Can you work these out from the model? Positions are in its coordinate system, mm. A direction names the side the tool comes from. Coordinates: 2 decimals unless noted, no trailing zeros. Order: outer loops, then holes, each group sorted by start corner. A loop starts at its lowest first (then second) coordinate and runs counter-clockwise, first axis right, second up. Notation, with made-up numbers: (26.25, -22) - (55.25, -22) arc R34 ccw to (55.25, 8) - close; hole circle Ø4 at (82.25, -21.5). An arc over 180 degrees is marked (long way). Return JSON: item names as keys, results as strings. Group by question number.
1) Imagine slicing it at C-C (y = -4.75). Write out the boundary of the cut face in (x, z), and give its area (3 significant figures).
2) If I drill on line 1 along Y through (x, z) = (-5.25, -5.5); line 2 along Z through (x, y) = (0, -2.75); line 3 along X through (y, z) = (-4.75, -1.75), over which ranges is the centre line in solid material (lowest first)?
3) If we mould it in two halves opening along X, with no side actions, what happens to faces 4 (the face through (9.4, 1.93, -0.11)), 5 (the face through (-9.43, 1.9, -0.11)), 6 (the face through (-7.5, -1, 0))? For each: pulls with the +X half, pulls with the -X half, needs draft (parallel to the pull), parting line crosses it, or undercut.
4) Imagine slicing it at B-B (x = 1.25). Write out the boundary of the cut face in (y, z).
5) Imagine slicing it at D-D (z = 1.75). Write out the boundary of the cut face in (x, y), and give its area (3 significant figures).
6) Which directions (+Z, -Z, +X, -X, +Y, -Y) give clear straight access to the entire face, cutting with the end or side of a thin tool? Please do faces 1 (the face through (-1, -3, -1.5)), 2 (the face through (1.5, -3, 1)), 3 (the face through (1, -3, -1.5)).
7) For pin 1 Ø2.5 at (y, z) = (-1.5, 0.5) entering from +X; pin 2 Ø0.5 at (x, y) = (1.5, -4.5) entering from +Z; pin 3 Ø0.5 at (y, z) = (-4, 1.5) entering from -X, each with a flat end and sliding along its axis, tell me the tip position at first contact or that it passes through.
8) Imagine slicing it at A-A (y = -1.5). Write out the boundary of the cut face in (x, z), and give its area (3 significant figures).
```python
from build123d import *

# Parameters (mm, degrees)
SKETCH1_W           = 20
SKETCH1_H           = 20
BOSS_EXTRUDE1_DEPTH = 2.5
BOSS_EXTRUDE2_DEPTH = 6
SKETCH3_W           = 2
SKETCH3_H           = 5
BOSS_EXTRUDE3_DEPTH = 3
FILLET1_R           = 2


with BuildPart() as part:
    # Sketch1 → Boss-Extrude1 (new body)
    with BuildSketch(Plane(origin=(0, 2.5, 0), x_dir=(1, 0, 0), z_dir=(0, 1, 0))):
        Rectangle(SKETCH1_W, SKETCH1_H)
    extrude(amount=-BOSS_EXTRUDE1_DEPTH)

    # Sketch2 → Boss-Extrude2 (add)
    with BuildSketch(Plane.XZ):
        with BuildLine():
            Line((-2.015564435, 1.000000009), (-1.000000005, 1.000000009))
            Line((-1.000000005, 1.000000009), (-1.000000005, 2.015564439))
            ThreePointArc((-1.000000005, 2.015564439), (0, 2.250000005), (1.000000005, 2.015564439))
            Line((1.000000005, 2.015564439), (1.000000005, 1.000000009))
            Line((1.000000005, 1.000000009), (2.015564435, 1.000000009))
            ThreePointArc((2.015564435, 1.000000009), (2.25, 5e-09), (2.015564435, -1))
            Line((2.015564435, -1), (1.000000005, -1))
            Line((1.000000005, -1), (1.000000005, -2.01556443))
            ThreePointArc((1.000000005, -2.01556443), (0, -2.249999995), (-1.000000005, -2.01556443))
            Line((-1.000000005, -2.01556443), (-1.000000005, -1))
            Line((-1.000000005, -1), (-2.015564435, -1))
            ThreePointArc((-2.015564435, -1), (-2.25, 5e-09), (-2.015564435, 1.000000009))
        make_face()
    extrude(amount=BOSS_EXTRUDE2_DEPTH)

    # Sketch3 → Boss-Extrude3 (add)
    with BuildSketch(Plane.XZ):
        with Locations((-8.5, 0)):
            Rectangle(SKETCH3_W, SKETCH3_H)
    extrude(amount=BOSS_EXTRUDE3_DEPTH)

    # Fillet1
    fillet1_edges = [part.edges().sort_by_distance(p)[0] for p in [
        (0, 2.5, 10),
        (-10, 2.5, 0),
        (0, 2.5, -10),
        (10, 2.5, 0),
        (10, 1.25, 10),
        (-10, 1.25, 10),
        (-10, 1.25, -10),
        (10, 1.25, -10),
    ]]
    fillet(fillet1_edges, radius=FILLET1_R)


solid = part.part
```
Calculated:
{
 "1": {"outline": "(-2.02, -1) - (-1, -1) - (-1, -2.02) arc R2.25 ccw to (1, -2.02) - (1, -1) - (2.02, -1) arc R2.25 ccw to (2.02, 1) - (1, 1) - (1, 2.02) arc R2.25 ccw to (-1, 2.02) - (-1, 1) - (-2.02, 1) arc R2.25 ccw to start", "area": "13.4 mm2"},
 "2": {"line 1": "0 to 2.5", "line 2": "-2.25 to 2.25", "line 3": "-1 to 1"},
 "3": {"face 4": "pulls with the +X half", "face 5": "pulls with the -X half", "face 6": "undercut"},
 "4": {"outline": "(-6, -1) - (0, -1) - (0, -10) - (0.5, -10) arc R2 ccw to (2.5, -8) - (2.5, 8) arc R2 ccw to (0.5, 10) - (0, 10) - (0, 1) - (-6, 1) - close"},
 "5": {"outline": "(-10, 0) - (-9.5, 0) - (-9.5, -3) - (-7.5, -3) - (-7.5, 0) - (-1, 0) - (-1, -6) - (1, -6) - (1, 0) - (10, 0) - (10, 0.5) arc R2 ccw to (8, 2.5) - (-8, 2.5) arc R2 ccw to (-10, 0.5) - close", "area": "66.3 mm2"},
 "6": {"face 1": "-Z, -Y", "face 2": "+Z, +X, -Y", "face 3": "-Z, +X, -Y"},
 "7": {"pin 1": "x = 2.25", "pin 2": "z = 1", "pin 3": "x = -1"},
 "8": {"outline": "(-9.5, -2.5) - (-7.5, -2.5) - (-7.5, 2.5) - (-9.5, 2.5) - close; (-2.02, -1) - (-1, -1) - (-1, -2.02) arc R2.25 ccw to (1, -2.02) - (1, -1) - (2.02, -1) arc R2.25 ccw to (2.02, 1) - (1, 1) - (1, 2.02) arc R2.25 ccw to (-1, 2.02) - (-1, 1) - (-2.02, 1) arc R2.25 ccw to start", "area": "23.4 mm2"}
}
